Geometry check sheet. Reference: the model listing, model coordinates, mm. Round coordinates to 2 decimals unless told otherwise and drop trailing zeros. Loops run counter-clockwise (first coordinate to the right, second up) from the corner with the lowest first, then second, coordinate; pieces in that order, holes last. Notation, with made-up numbers: (-14.5, -9) - (26.5, -9) arc R17 ccw to (26.5, 14) - close; hole circle Ø6 at (68.25, -20). An arc over 180 degrees is marked (long way). Answer in a Markdown table with one row per item. Add a question column.
```python
from build123d import *

# Parameters (mm, degrees)
BOSS_EXTRUDE1_DEPTH = 5
SKETCH4_W           = 5
SKETCH4_H           = 85
CUT_EXTRUDE3_DEPTH  = 6
CUT_EXTRUDE6_DEPTH  = 6
CUT_EXTRUDE8_DEPTH  = 5
SKETCH10_R          = 2.1
SKETCH10_W          = 50
SKETCH10_H          = 5
SKETCH10_W_2        = 15
SKETCH10_H_2        = 30
CUT_EXTRUDE9_DEPTH  = 10
CUT_EXTRUDE10_DEPTH = 10


with BuildPart() as part:
    # Sketch1 → Boss-Extrude1 (new body)
    with BuildSketch(Plane.XY):
        Polygon((64.226162893, -107), (118, -107), (118, 83), (98, 103), (-98, 103), (-118, 83), (-118, -107), (-64.226162893, -107), align=None)
    extrude(amount=BOSS_EXTRUDE1_DEPTH)

    # Sketch4 → Cut-Extrude3 (cut, through all)
    with BuildSketch(Plane.XY.offset(5)):
        with Locations((-115.5, -2)):
            Rectangle(SKETCH4_W, SKETCH4_H)
        with Locations((115.5, -2)):
            Rectangle(SKETCH4_W, SKETCH4_H)
    extrude(amount=-CUT_EXTRUDE3_DEPTH, mode=Mode.SUBTRACT)

    # Sketch7 → Cut-Extrude6 (cut, through all)
    with BuildSketch(Plane.XY.offset(5)):
        Polygon((-15, 98), (-2.4, 98), (-2.4, 94), (-4.4, 94), (-4.4, 91.2), (-2.4, 91.2), (-2.4, 85.2), (2.4, 85.2), (2.4, 91.2), (4.4, 91.2), (4.4, 94), (2.4, 94), (2.4, 98), (15, 98), (15, 103), (-15, 103), align=None)
        Polygon((-51.315063509, 98), (-63.915063509, 98), (-63.915063509, 103), (-33.915063509, 103), (-33.915063509, 98), (-46.515063509, 98), (-46.515063509, 94), (-44.515063509, 94), (-44.515063509, 91.2), (-46.515063509, 91.2), (-46.515063509, 85.2), (-51.315063509, 85.2), (-51.315063509, 91.2), (-53.315063509, 91.2), (-53.315063509, 94), (-51.315063509, 94), align=None)
        Polygon((-102.765899705, 91.163032483), (-99.93747258, 88.334605358), (-98.523259018, 89.748818921), (-96.543360031, 87.768919933), (-97.957573593, 86.354706371), (-93.714932906, 82.112065684), (-97.109045456, 78.717953134), (-101.351686143, 82.960593821), (-102.765899705, 81.546380259), (-104.745798693, 83.526279246), (-103.33158513, 84.940492808), (-106.160012255, 87.768919933), align=None)
        Polygon((93.714932906, 82.112065684), (97.109045456, 78.717953134), (101.351686143, 82.960593821), (102.765899705, 81.546380259), (104.745798693, 83.526279246), (103.33158513, 84.940492808), (106.160012255, 87.768919933), (102.765899705, 91.163032483), (99.93747258, 88.334605358), (98.523259018, 89.748818921), (96.543360031, 87.768919933), (97.957573593, 86.354706371), align=None)
        Polygon((33.915063509, 98), (46.515063509, 98), (46.515063509, 94), (44.515063509, 94), (44.515063509, 91.2), (46.515063509, 91.2), (46.515063509, 85.2), (51.315063509, 85.2), (51.315063509, 91.2), (53.315063509, 91.2), (53.315063509, 94), (51.315063509, 94), (51.315063509, 98), (63.915063509, 98), (63.915063509, 103), (33.915063509, 103), align=None)
    extrude(amount=-CUT_EXTRUDE6_DEPTH, mode=Mode.SUBTRACT)

    # Sketch9 → Cut-Extrude8 (cut)
    with BuildSketch(Plane.XY.offset(5)):
        Polygon((94.467486322, 99.461445866), (98, 103), (118, 83), (114.464466094, 79.464466094), align=None)
        Polygon((-118, 83), (-114.461445866, 79.467486322), (-94.464466094, 99.464466094), (-98, 103), align=None)
    extrude(amount=-CUT_EXTRUDE8_DEPTH, mode=Mode.SUBTRACT)

    # Sketch10 → Cut-Extrude9 (cut)
    with BuildSketch(Plane.XY.offset(5)):
        with Locations((69, 42.5)):
            Circle(SKETCH10_R)
        with Locations((-69, 42.5)):
            Circle(SKETCH10_R)
        with Locations((0, 42.5)):
            Rectangle(SKETCH10_W, SKETCH10_H)
        with Locations((-69, 67.5)):
            Rectangle(SKETCH10_W_2, SKETCH10_H_2)
        with Locations((0, 67.5)):
            Rectangle(SKETCH10_W_2, SKETCH10_H_2)
        with Locations((69, 67.5)):
            Rectangle(SKETCH10_W_2, SKETCH10_H_2)
        with BuildLine():
            Line((-54, 82.5), (-54, 52.5))
            ThreePointArc((-54, 52.5), (-56.5, 50), (-59, 52.5))
            Line((-59, 52.5), (-59, 82.5))
            ThreePointArc((-59, 82.5), (-56.5, 85), (-54, 82.5))
        make_face()
        with BuildLine():
            Line((-9, 82.5), (-9, 52.5))
            ThreePointArc((-9, 52.5), (-11.5, 50), (-14, 52.5))
            Line((-14, 52.5), (-14, 82.5))
            ThreePointArc((-14, 82.5), (-11.5, 85), (-9, 82.5))
        make_face()
        with BuildLine():
            Line((58.5, 82.5), (58.5, 52.5))
            ThreePointArc((58.5, 52.5), (56, 50), (53.5, 52.5))
            Line((53.5, 52.5), (53.5, 82.5))
            ThreePointArc((53.5, 82.5), (56, 85), (58.5, 82.5))
        make_face()
        with BuildLine():
            Line((-84, 82.5), (-84, 52.5))
            ThreePointArc((-84, 52.5), (-81.5, 50), (-79, 52.5))
            Line((-79, 52.5), (-79, 82.5))
            ThreePointArc((-79, 82.5), (-81.5, 85), (-84, 82.5))
        make_face()
        with BuildLine():
            Line((9, 82.5), (9, 52.5))
            ThreePointArc((9, 52.5), (11.5, 50), (14, 52.5))
            Line((14, 52.5), (14, 82.5))
            ThreePointArc((14, 82.5), (11.5, 85), (9, 82.5))
        make_face()
        with BuildLine():
            Line((79.5, 82.5), (79.5, 52.5))
            ThreePointArc((79.5, 52.5), (82, 50), (84.5, 52.5))
            Line((84.5, 52.5), (84.5, 82.5))
            ThreePointArc((84.5, 82.5), (82, 85), (79.5, 82.5))
        make_face()
    extrude(amount=-CUT_EXTRUDE9_DEPTH, mode=Mode.SUBTRACT)

    # Sketch11 → Cut-Extrude10 (cut)
    with BuildSketch(Plane.XY.offset(5)):
        Polygon((-113, 0.4), (-109, 0.4), (-109, 2.4), (-106.2, 2.4), (-106.2, 0.4), (-100.2, 0.4), (-100.2, -4.4), (-106.2, -4.4), (-106.2, -6.4), (-109, -6.4), (-109, -4.4), (-113, -4.4), align=None)
        Polygon((113, 0.4), (113, -4.4), (109, -4.4), (109, -6.4), (106.2, -6.4), (106.2, -4.4), (100.2, -4.4), (100.2, 0.4), (106.2, 0.4), (106.2, 2.4), (109, 2.4), (109, 0.4), align=None)
    extrude(amount=-CUT_EXTRUDE10_DEPTH, mode=Mode.SUBTRACT)


solid = part.part
```
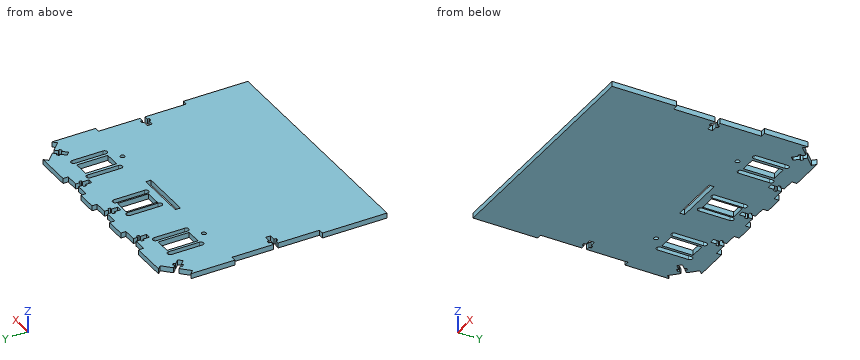
Q1. Depth check by flat-ended pin: P1, Ø0.6, axis at x = -52, z = 2, coming from the +Y side; P2, Ø2.5, axis at x = -114.5, z = 1.5, coming from the +Y side; P3, Ø1.5, axis at y = 99.5, z = 3, coming from the +X side. Enter the tip coordinate at first touch or a pass-through.
Q2. Cross-section at C-C, the plane y = 8. Enter the section's corners in (x, z).
Q3. Scan lines: line 1 (X direction, y = 1, z = 4.1); line 2 (Y direction, x = -69, z = 2.9); line 3 (Y direction, x = 5, z = 2.3). Record each from-to range of solid material in increasing order. Write a range as from..to.
Q4. Cross-section at A-A, the plane y = 68.5. State how many separate pieces and enclosed holes the cut face has, plus the area to 3 significant figures.
Check sheet entries:
| question | item | result |
|---|---|---|
| 1 | P1 | y = 98 |
| 1 | P2 | y = 80.75 |
| 1 | P3 | x = 95.25 |
| 2 | outline | (-113, 0) - (113, 0) - (113, 5) - (-113, 5) - close |
| 3 | line 1 | -113..-109, -106.2..106.2, 109..113 |
| 3 | line 2 | -107..40.4, 44.6..52.5, 82.5..103 |
| 3 | line 3 | -107..40, 45..52.5, 82.5..98 |
| 4 | separate pieces | 10 |
| 4 | enclosed holes | 0 |
| 4 | area | 805 mm² |
